Verification items for the finished model (mm, model axes). Round coordinates to 2 decimals unless told otherwise and drop trailing zeros. Write each loop counter-clockwise with the first axis right and the second up, starting at its lowest first coordinate (ties: lowest second). Pieces come first, ordered by that corner, then holes. Notation, with made-up numbers: M 83,60 L 110,60 A29 cw 110,86 Z; hole C 12,73 d10. An arc over 180 degrees is marked long. One line per question, with ' | ' between items.
from build123d import *

# Parameters (mm, degrees)
F0_R     = 38.1
F1_DEPTH = 488.95
F4_DEPTH = 10.7442


# Not quite as in the source:
# - a pattern or mirror of a feature is missing from the dataset's text; its kind, count and spacing are read off the source's solid


with BuildPart() as f1:
    # F0 (on Front) → F1 (new body, symmetric)
    with BuildSketch(Plane.XZ):
        Circle(F0_R)
    extrude(amount=F1_DEPTH, both=True)

    # F3 (on offset) → F4 (cut)
    with BuildSketch(Plane.XY.offset(38.1)):
        with BuildLine():
            Line((-9.525, -361.95), (-9.525, -574.1807818413))
            Line((-9.525, -574.1807818413), (9.525, -574.1807818413))
            Line((9.525, -574.1807818413), (9.525, -361.95))
            ThreePointArc((9.525, -361.95), (0, -352.425), (-9.525, -361.95))
        make_face()
    f4 = extrude(amount=-F4_DEPTH, mode=Mode.SUBTRACT)

    # F4_copies: F4 across plane
    add(f4.mirror(Plane.ZX), mode=Mode.SUBTRACT)


solid = f1.part
1. Go/stop test with flat-tipped pins: P1, Ø12, axis at y = -295.5, z = -19.5, coming from the +X side; P2, Ø1, axis at y = -337.5, z = 12, coming from the -X side; P3, Ø10.5, axis at y = 397, z = 33.5, coming from the +X side. Record where each tip stops, or that it passes through.
Results:
P1: stops at x = 35.63 | P2: stops at x = -36.32 | P3: stops at x = 25.56
2. Section check B-B, the plane y = 306. Record the cut outline in (x, z).
Results:
outline: C 0,0 d76.2
3. Thickness scan on line 1 (X direction, y = 219, z = -3); line 2 (X direction, y = 308.5, z = 28); line 3 (Z direction, x = 20.5, y = 376). Record the ranges inside material, lowest first.
Results:
line 1: x = -37.98 to 37.98 | line 2: x = -25.84 to 25.84 | line 3: z = -32.11 to 32.11
4. Section check C-C, the plane z = -27. Record the cut outline in (x, y), then the cut area to 3 significant figures.
Results:
outline: M -26.88,-488.95 L 26.88,-488.95 L 26.88,488.95 L -26.88,488.95 Z | area: 52,600 mm2
5. Mould release check, pull along X, two halves, no side actions. Record for faces 1 (the face through (0, 420, 27.356)), 2 (the face through (-1, -488.95, 0)), 3 (the face through (-8.259, -6.845, -37.194)), 4 (the face through (0, -420, 27.356)): pulls with the +X half, pulls with the -X half, needs draft (parallel to the pull), parting line crosses it, or undercut.
Results:
face 1: undercut | face 2: needs draft | face 3: parting line crosses it | face 4: undercut
6. Section check A-A, the plane x = 0. Record the cut outline in (y, z) (3 decimals), then the cut area to 3 significant figures.
Results:
outline: M -488.95,-38.1 L 488.95,-38.1 L 488.95,27.356 L 352.425,27.356 L 352.425,38.1 L -352.425,38.1 L -352.425,27.356 L -488.95,27.356 Z | area: 71,600 mm2
